Geometry check sheet. Reference: the model listing, model coordinates, mm. A direction names the side the tool comes from. Round coordinates to 2 decimals unless told otherwise and drop trailing zeros. Loops run counter-clockwise (first coordinate to the right, second up) from the corner with the lowest first, then second, coordinate; pieces in that order, holes last. Notation, with made-up numbers: (72, 42) -> (110, 42) arc R16 cw to (110, 70) -> close; hole circle Ø11 at (79.25, 1.25). An arc over 180 degrees is marked (long way). Use one line per item in the form item = value.
from build123d import *

# Parameters (mm, degrees)
F0_W     = 101.6
F0_H     = 50.8
F1_DEPTH = 25.4
F3_R     = 12.626105
F4_DEPTH = 50.8
F5_D     = 6.35


with BuildPart() as f1:
    # F0 (on Top) → F1 (new body)
    with BuildSketch(Plane.XY):
        with Locations((0, 2.451474)):
            Rectangle(F0_W, F0_H)
    extrude(amount=F1_DEPTH)

    # F3 (on face) → F4 (join)
    with BuildSketch(Plane.XY.offset(25.4)):
        Circle(F3_R)
    extrude(amount=F4_DEPTH)

    # F5 (through all)
    with Locations(Plane.XY.offset(25.4)):
        with Locations((-41.046023, -13.491523), (39.856285, -13.491523), (39.856285, 18.040607), (-41.640893, 18.33808)):
            Hole(F5_D / 2)


solid = f1.part
1. Section check A-A (x = 0). Record the boundary of the cut face in (y, z), then the cut area to 3 significant figures.
Return value:
outline = (-22.95, 0) -> (27.85, 0) -> (27.85, 25.4) -> (12.63, 25.4) -> (12.63, 76.2) -> (-12.63, 76.2) -> (-12.63, 25.4) -> (-22.95, 25.4) -> close
area = 2,570 mm2
2. Section check C-C (y = 16.5). Record the boundary of the cut face in (x, z).
Return value:
outline = (-50.8, 0) -> (-44.23, 0) -> (-44.23, 25.4) -> (-50.8, 25.4) -> close; (-39.05, 0) -> (37.08, 0) -> (37.08, 25.4) -> (-39.05, 25.4) -> close; (42.63, 0) -> (50.8, 0) -> (50.8, 25.4) -> (42.63, 25.4) -> close
3. Section check D-D (z = 65). Record the boundary of the cut face in (x, y), then the cut area to 3 significant figures.
Return value:
outline = circle Ø25.25 at (0, 0)
area = 501 mm2
4. Mould release check, pull along Y, two halves, no side actions. Record for faces 1 (the flat face through (-1, 14, 25.4)), 2 (the flat face through (-1, 27.851, 13)), 3 (the cylindrical face through (-44.67, 19.29, 12.52)): released by +Y, released by -Y, zero draft, split by the parting line, or undercut.
Return value:
face_1 = zero draft
face_2 = released by +Y
face_3 = undercut
5. Material ranges on line 1 along X through (y, z) = (-11, 5); line 2 along X through (y, z) = (20.5, 17.5); line 3 along Z through (x, y) = (22, 6.5), recorded low to high.
Return value:
line_1 = -50.8 to -43.01, -39.08 to 37.89, 41.82 to 50.8
line_2 = -50.8 to -43.97, -39.32 to 37.85, 41.86 to 50.8
line_3 = 0 to 25.4
6. Section check B-B (y = 0). Record the boundary of the cut face in (x, z), then the cut area to 3 significant figures.
Return value:
outline = (-50.8, 0) -> (50.8, 0) -> (50.8, 25.4) -> (12.63, 25.4) -> (12.63, 76.2) -> (-12.63, 76.2) -> (-12.63, 25.4) -> (-50.8, 25.4) -> close
area = 3,860 mm2
7. Tool access check on faces 4 (the flat face through (0, 0, 76.2)), 5 (the cylindrical face through (12.043, 3.793, 50.444)). Record the directions out of +Z, -Z, +X, -X, +Y, -Y that give a thin tool (end or side, any length) a straight path to the whole face; none if there is none.
Return value:
face_4 = +Z, +X, -X, +Y, -Y
face_5 = +Z
8. Gauge pin test, flat ends, axial feed: pin 1 (3 mm diameter, centred on y = -2.5, z = 63, fed in from +X); pin 2 (1.5 mm diameter, centred on x = 32.5, y = 8, fed in from +Z); pin 3 (6 mm diameter, centred on y = -6.5, z = 66.5, fed in from +X). Record the tip position at first contact, or that the pin passes through.
Return value:
pin_1 = 12.59
pin_2 = 25.4
pin_3 = 12.13
